Geometry: final body of the model. Coordinates: model frame, mm. Face numbers are marked on the shaded views. A direction names the side the tool comes from. Coordinates: 2 decimals unless noted, no trailing zeros. Write each loop counter-clockwise with the first axis right and the second up, starting at its lowest first coordinate (ties: lowest second). Pieces come first, ordered by that corner, then holes.
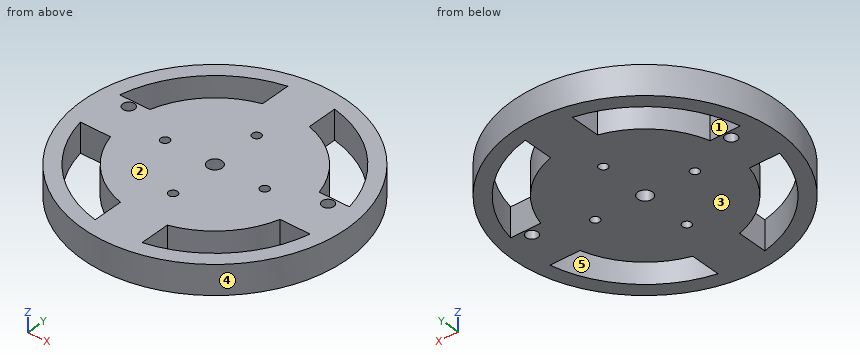
from build123d import *

# Parameters (mm, degrees)
SKETCH1_R           = 45
SKETCH1_R_2         = 2.5
SKETCH1_R_3         = 1.5
BOSS_EXTRUDE1_DEPTH = 10
SKETCH3_R           = 2
CUT_EXTRUDE1_DEPTH  = 10


with BuildPart() as part:
    # Sketch1 → Boss-Extrude1 (new body)
    with BuildSketch(Plane.XY):
        Circle(SKETCH1_R)
        Circle(SKETCH1_R_2, mode=Mode.SUBTRACT)
        with Locations((0, 17)):
            Circle(SKETCH1_R_3, mode=Mode.SUBTRACT)
        with Locations((17, 0)):
            Circle(SKETCH1_R_3, mode=Mode.SUBTRACT)
        with Locations((0, -17)):
            Circle(SKETCH1_R_3, mode=Mode.SUBTRACT)
        with Locations((-17, 0)):
            Circle(SKETCH1_R_3, mode=Mode.SUBTRACT)
        with BuildLine():
            Line((28.91366459, 8), (39.191835885, 8))
            ThreePointArc((39.191835885, 8), (28.284271247, 28.284271247), (8, 39.191835885))
            Line((8, 39.191835885), (8, 28.91366459))
            ThreePointArc((8, 28.91366459), (21.213203436, 21.213203436), (28.91366459, 8))
        make_face(mode=Mode.SUBTRACT)
        with BuildLine():
            Line((28.91366459, -8), (39.191835885, -8))
            ThreePointArc((39.191835885, -8), (28.284271247, -28.284271247), (8, -39.191835885))
            Line((8, -39.191835885), (8, -28.91366459))
            ThreePointArc((8, -28.91366459), (21.213203436, -21.213203436), (28.91366459, -8))
        make_face(mode=Mode.SUBTRACT)
        with BuildLine():
            Line((-8, -28.91366459), (-8, -39.191835885))
            ThreePointArc((-8, -39.191835885), (-28.284271247, -28.284271247), (-39.191835885, -8))
            Line((-39.191835885, -8), (-28.91366459, -8))
            ThreePointArc((-28.91366459, -8), (-21.213203436, -21.213203436), (-8, -28.91366459))
        make_face(mode=Mode.SUBTRACT)
        with BuildLine():
            Line((-39.191835885, 8), (-28.91366459, 8))
            ThreePointArc((-28.91366459, 8), (-21.213203436, 21.213203436), (-8, 28.91366459))
            Line((-8, 28.91366459), (-8, 39.191835885))
            ThreePointArc((-8, 39.191835885), (-28.284271247, 28.284271247), (-39.191835885, 8))
        make_face(mode=Mode.SUBTRACT)
    extrude(amount=BOSS_EXTRUDE1_DEPTH)

    # Sketch3 → Cut-Extrude1 (cut)
    with BuildSketch(Plane.XY.offset(10)):
        with Locations((-34, 5.5)):
            Circle(SKETCH3_R)
        with Locations((34, 5.5)):
            Circle(SKETCH3_R)
    extrude(amount=-CUT_EXTRUDE1_DEPTH, mode=Mode.SUBTRACT)


solid = part.part
Item 1: Section C-C, the plane z = 5. State how many separate pieces and enclosed holes the cut face has, plus the area to 3 significant figures.
Derived:
separate pieces: 1
enclosed holes: 11
area: 4,740 mm2
Item 2: Set-up query: the marked faces 1 and 2. Return all of +Z, -Z, +X, -X, +Y, -Y with unobstructed straight access to the full face (end or side cutting, diameter ignored); none if empty.
Derived:
face 1: +Z, -Z
face 2: +Z, +X, -X, +Y, -Y
Item 3: Section D-D, the plane y = 32.5. Output: boundary loops of the cut face in (x, z), plus the area to 3 significant figures.
Derived:
outline: (-31.12, 0) - (-23.32, 0) - (-23.32, 10) - (-31.12, 10) - close; (-8, 0) - (8, 0) - (8, 10) - (-8, 10) - close; (23.32, 0) - (31.12, 0) - (31.12, 10) - (23.32, 10) - close
area: 316 mm2
Item 4: Pin query (flat end, axial travel): pin 1 (4 mm diameter, centred on x = 11, z = 3.5, fed in from +Y); pin 2 (4 mm diameter, centred on y = 3, z = 4, fed in from -X); pin 3 (3 mm diameter, centred on x = -33, z = 6, fed in from +Y); pin 4 (3.5 mm diameter, centred on x = 34, y = 5.5, fed in from -Z). Return the tip coordinate at first contact, or that it passes through.
Derived:
pin 1: stops at y = 44.09
pin 2: stops at x = -44.99
pin 3: stops at y = 32.14
pin 4: passes through
Item 5: Material intervals for probe 1 along Y at (x, z) = (0, 3); probe 2 along Y at (x, z) = (17, 4.5); probe 3 along Y at (x, z) = (15, 4.75), sorted ascending.
Derived:
probe 1: y = -45 to -18.5, -15.5 to -2.5, 2.5 to 15.5, 18.5 to 45
probe 2: y = -41.67 to -36.21, -24.72 to -1.5, 1.5 to 24.72, 36.21 to 41.67
probe 3: y = -42.43 to -37.08, -25.98 to 25.98, 37.08 to 42.43
Item 6: Pull-direction query (Y, two-part tool) for the marked faces 3, 4 and 5; classes: released by +Y, released by -Y, zero draft, split by the parting line, or undercut.
Derived:
face 3: zero draft
face 4: split by the parting line
face 5: undercut
Item 7: Section A-A, the plane y = 0. Output: boundary loops of the cut face in (x, z), plus the area to 3 significant figures.
Derived:
outline: (-45, 0) - (-18.5, 0) - (-18.5, 10) - (-45, 10) - close; (-15.5, 0) - (-2.5, 0) - (-2.5, 10) - (-15.5, 10) - close; (2.5, 0) - (15.5, 0) - (15.5, 10) - (2.5, 10) - close; (18.5, 0) - (45, 0) - (45, 10) - (18.5, 10) - close
area: 790 mm2
Item 8: Section B-B, the plane x = -34. Output: boundary loops of the cut face in (y, z), plus the area to 3 significant figures.
Derived:
outline: (-29.48, 0) - (-21.07, 0) - (-21.07, 10) - (-29.48, 10) - close; (-8, 0) - (3.5, 0) - (3.5, 10) - (-8, 10) - close; (7.5, 0) - (8, 0) - (8, 10) - (7.5, 10) - close; (21.07, 0) - (29.48, 0) - (29.48, 10) - (21.07, 10) - close
area: 288 mm2
